Verification items for the finished model (mm, model axes). Face numbers are marked on the shaded views. A direction names the side the tool comes from. Give positions to 0.01 mm unless a question says otherwise; leave off trailing zeros. Loops run counter-clockwise (first coordinate to the right, second up) from the corner with the lowest first, then second, coordinate; pieces in that order, holes last. Notation, with made-up numbers: M 3.5,20 L 30.5,20 A22 cw 30.5,44 Z; hole C -20.5,-39.75 d1. An arc over 180 degrees is marked long. Put each result on its own line as item: value. Start each with the question number.
from build123d import *

# Parameters (mm, degrees)
SKETCH1_R               = 15.875
BOSS_EXTRUDE1_DEPTH     = 12.7
F_3_8_CLEARANCE_HOLE1_D = 10.31748
CUT_EXTRUDE1_DEPTH      = 26.793821935
CUT_EXTRUDE1_DEPTH_BACK = 26.793821935
SKETCH4_R               = 1.5875


with BuildPart() as part:
    # Sketch1 → Boss-Extrude1 (new body)
    with BuildSketch(Plane(origin=(0, 0, 0), x_dir=(1, 0, 0), z_dir=(0, 1, 0))):
        with Locations(Location((0, 0, 0), (0, 0, 270))):
            Circle(SKETCH1_R)
    extrude(amount=BOSS_EXTRUDE1_DEPTH)

    # 3/8 Clearance Hole1 (through all)
    with Locations(Plane(origin=(0, 12.7, 0), x_dir=(1, 0, 0), z_dir=(0, 1, 0))):
        with Locations((0, 0)):
            Hole(F_3_8_CLEARANCE_HOLE1_D / 2)


with BuildPart() as body_2:
    # uxcell-FR6ZZ: read off the stored shape, not the designer's step
    # uxcell-FR6ZZ outline → uxcell-FR6ZZ (revolve)
    with BuildSketch(Plane(origin=(-41.000177455, 0, 16.423895222), x_dir=(1, 0, 0), z_dir=(0, 0, 1))):
        Polygon((12.303125, 21.164419461), (4.7625, 21.164419461), (4.7625, 14.020669461), (11.1125, 14.020669461), (11.1125, 19.180044461), (11.509375, 19.576919461), (12.303125, 19.576919461), align=None)
    revolve(axis=Axis((-41.000177455, 0, 16.423895222), (0, 1, 0)))


with BuildPart() as body_2_1:
    # Body-Move/Copy2: read off the stored shape, not the designer's step
    # Body-Move/Copy2: moved
    add(body_2.part.moved(Location((41.0001775, -8.4644195, -16.4238952))))


with BuildPart() as part_1:
    add(part.part)

    # Combine1: cut body 2
    add(body_2_1.part, mode=Mode.SUBTRACT)

    # Sketch4 → Cut-Extrude1 (cut, two sides: drawn at the far end of the back side and taken through both)
    with BuildSketch(Plane(origin=(0, 0, 0), x_dir=(1, 0, 0), z_dir=(0, 1, 0)).offset(-CUT_EXTRUDE1_DEPTH_BACK)):
        with Locations(Location((-8.96874, 0, 0), (0, 0, 270))):
            Circle(SKETCH4_R)
        with Locations(Location((8.96874, 0, 0), (0, 0, 270))):
            Circle(SKETCH4_R)
    extrude(amount=CUT_EXTRUDE1_DEPTH + CUT_EXTRUDE1_DEPTH_BACK, mode=Mode.SUBTRACT)


solid = part_1.part
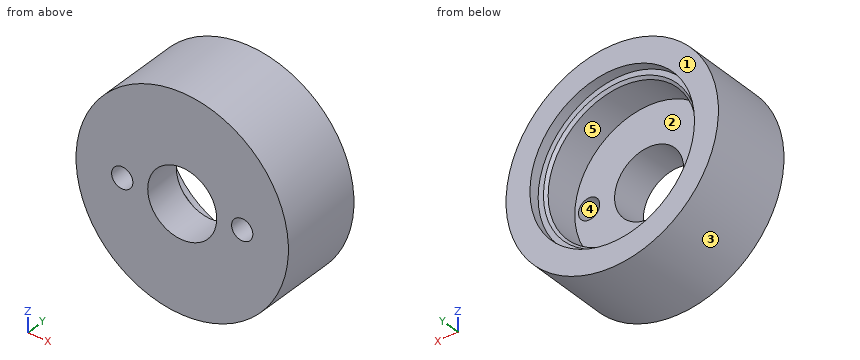
Q1. Set-up check for the marked faces 4 and 5: record each of +Z, -Z, +X, -X, +Y, -Y from which the full face is reachable in a straight line by a thin tool's end or side.
Q2. Go/stop test with flat-tipped pins: pin 1 (4 mm diameter, centred on y = 11.5, z = -0.5, fed in from +X) (3 decimals); pin 2 (13.5 mm diameter, centred on x = 0, z = 0, fed in from +Y); pin 3 (1.5 mm diameter, centred on x = 8, y = 9, fed in from +Z); pin 4 (4 mm diameter, centred on y = 4.5, z = 5.5, fed in from -X). Record where each tip stops, or that it passes through.
Q3. Release check for a two-part mould opening along Z. For the marked faces 1, 2 and 3 record: pulls with the +Z half, pulls with the -Z half, needs draft (parallel to the pull), parting line crosses it, or undercut.
Q4. Scan lines: L1, parallel to Y at x = -6, z = 0; L2, parallel to Z at x = 9, y = 11; L3, parallel to X at y = 4.5, z = -4.5. Record each from-to range of solid material in increasing order.
Q5. Cross-section at A-A, the plane x = 0. Record the boundary of the cut face in (y, z) (1 decimal), then the cut area to 3 significant figures.
Q6. Cross-section at B-B, the plane z = 0. Record the boundary of the cut face in (x, y) (1 decimal), then the cut area to 3 significant figures.
Ans:
1. face 4: +Y, -Y
1. face 5: +Y
2. pin 1: stops at x = 15.875
2. pin 2: stops at y = 5.56
2. pin 3: stops at z = 14.12
2. pin 4: stops at x = -15.48
3. face 1: needs draft
3. face 2: undercut
3. face 3: parting line crosses it
4. L1: y = 0 to 5.56
4. L2: z = -13.08 to -6.99, 6.99 to 13.08
4. L3: x = -15.22 to -2.52, 2.52 to 15.22
5. outline: M 0,-15.9 L 12.7,-15.9 L 12.7,-12.3 L 11.1,-12.3 L 11.1,-11.5 L 10.7,-11.1 L 5.6,-11.1 L 5.6,-5.2 L 0,-5.2 Z; M 0,5.2 L 5.6,5.2 L 5.6,11.1 L 10.7,11.1 L 11.1,11.5 L 11.1,12.3 L 12.7,12.3 L 12.7,15.9 L 0,15.9 Z
5. area: 183 mm^2
6. outline: M -15.9,0 L -10.6,0 L -10.6,5.6 L -11.1,5.6 L -11.1,10.7 L -11.5,11.1 L -12.3,11.1 L -12.3,12.7 L -15.9,12.7 Z; M -7.4,0 L -5.2,0 L -5.2,5.6 L -7.4,5.6 Z; M 5.2,0 L 7.4,0 L 7.4,5.6 L 5.2,5.6 Z; M 10.6,0 L 15.9,0 L 15.9,12.7 L 12.3,12.7 L 12.3,11.1 L 11.5,11.1 L 11.1,10.7 L 11.1,5.6 L 10.6,5.6 Z
6. area: 148 mm^2
